from build123d import *

# Parameters (mm, degrees)
SKETCH2_R           = 57.15
SKETCH2_R_2         = 50.8
BOSS_EXTRUDE1_DEPTH = 101.6
SKETCH4_R           = 57.15
SKETCH4_R_2         = 50.8
BOSS_EXTRUDE2_DEPTH = 1.016
SKETCH5_R           = 1.27
CUT_EXTRUDE2_DEPTH  = 14.732


with BuildPart() as part:
    # Sketch2 → Boss-Extrude1 (new body)
    with BuildSketch(Plane(origin=(0, 0, 0), x_dir=(1, 0, 0), z_dir=(0, 1, 0))):
        with Locations(Location((0, 0, 0), (0, 0, 270))):
            Circle(SKETCH2_R)
        with Locations(Location((0, 0, 0), (0, 0, 270))):
            Circle(SKETCH2_R_2, mode=Mode.SUBTRACT)
    extrude(amount=BOSS_EXTRUDE1_DEPTH)

    # Sketch4 → Boss-Extrude2 (add)
    # profile 1 of 2: a face of its own
    with BuildSketch(Plane(origin=(0, 101.6, 0), x_dir=(1, 0, 0), z_dir=(0, 1, 0))):
        with Locations(Location((0, 0, 0), (0, 0, 270))):
            Circle(SKETCH4_R)
        with Locations(Location((0, 0, 0), (0, 0, 172.649423361))):
            Circle(SKETCH4_R_2, mode=Mode.SUBTRACT)
    # profile 2 of 2: a face of its own
    with BuildSketch(Plane(origin=(0, 101.6, 0), x_dir=(1, 0, 0), z_dir=(0, 1, 0))):
        with BuildLine():
            Line((-50.382520142, -6.499358748), (0, -6.499358748))
            Line((0, -6.499358748), (50.382520142, -6.499358748))
            ThreePointArc((50.382520142, -6.499358748), (50.695522599, -3.256376574), (50.8, 0))
            ThreePointArc((50.8, 0), (50.695522599, 3.256376574), (50.382520142, 6.499358748))
            Line((50.382520142, 6.499358748), (-50.382520142, 6.499358748))
            ThreePointArc((-50.382520142, 6.499358748), (-50.8, 0), (-50.382520142, -6.499358748))
        make_face()
    extrude(amount=BOSS_EXTRUDE2_DEPTH)

    # Sketch5 → Cut-Extrude2 (cut)
    with BuildSketch(Plane(origin=(0, 102.616, 0), x_dir=(1, 0, 0), z_dir=(0, 1, 0))):
        with Locations(Location((7.62, 0, 0), (0, 0, 270))):
            Circle(SKETCH5_R)
        with Locations(Location((-7.62, 0, 0), (0, 0, 270))):
            Circle(SKETCH5_R)
    extrude(amount=-CUT_EXTRUDE2_DEPTH, mode=Mode.SUBTRACT)


solid = part.part
Work out the finished part from the listing and answer in its coordinate system (mm). Coordinates: 2 decimals unless noted, no trailing zeros. Loops run counter-clockwise (first coordinate to the right, second up) from the corner with the lowest first, then second, coordinate; pieces in that order, holes last. Notation, with made-up numbers: M 79,41 L 100,41 A27 ccw 100,60 Z; hole C 79,81.25 d10. An arc over 180 degrees is marked long. Answer in a Markdown table with one row per item. Add a question column.
1. Flat-ended cylindrical pins translate along their axes: P1, Ø0.5, axis at x = 8, y = 102, coming from the +Z side; P2, Ø1.5, axis at x = -25, y = 76, coming from the -Z side; P3, Ø4, axis at x = -8.5, y = 14, coming from the -Z side. Find the tip coordinate at first contact, or state that the pin passes through.
2. Find section B-B, the plane z = 20.5. Write down the section's boundary in (x, y), then the cut area to 3 significant figures.
3. Find section A-A, the plane x = 0. Write down the section's boundary in (y, z).
4. The mould has two halves that part along Z. Classify faces 1 (the flat face through (-1, 101.6, 0)), 2 (the cylindrical face through (2.513, 50.59, -57.095)), 3 (the flat face through (-4, 102.616, 0)): pulls with the +Z half, pulls with the -Z half, needs draft (parallel to the pull), parting line crosses it, or undercut.
5. Consider L1, parallel to X at y = 102, z = 0; L2, parallel to X at y = 56, z = 0; L3, parallel to Z at x = 1, y = 60.5. Determine where each line is inside the solid, lowest interval first.
6. Find section C-C, the plane y = 30. Write down the section's boundary in (x, z).
7. Find section D-D, the plane x = 20.5. Write down the section's boundary in (y, z).
Reported:
| question | item | result |
|---|---|---|
| 1 | P1 | stops at z = 56.62 |
| 1 | P2 | stops at z = -51.75 |
| 1 | P3 | stops at z = -56.78 |
| 2 | outline | M -53.35,0 L -46.48,0 L -46.48,102.62 L -53.35,102.62 Z; M 46.48,0 L 53.35,0 L 53.35,102.62 L 46.48,102.62 Z |
| 2 | area | 1,410 mm^2 |
| 3 | outline | M 0,-57.15 L 102.62,-57.15 L 102.62,-50.8 L 0,-50.8 Z; M 0,50.8 L 102.62,50.8 L 102.62,57.15 L 0,57.15 Z; M 101.6,-6.5 L 102.62,-6.5 L 102.62,6.5 L 101.6,6.5 Z |
| 4 | face 1 | undercut |
| 4 | face 2 | parting line crosses it |
| 4 | face 3 | needs draft |
| 5 | L1 | x = -57.15 to -8.89, -6.35 to 6.35, 8.89 to 57.15 |
| 5 | L2 | x = -57.15 to -50.8, 50.8 to 57.15 |
| 5 | L3 | z = -57.14 to -50.79, 50.79 to 57.14 |
| 6 | outline | C 0,0 d114.3; hole C 0,0 d101.6 |
| 7 | outline | M 0,-53.35 L 102.62,-53.35 L 102.62,-46.48 L 0,-46.48 Z; M 0,46.48 L 102.62,46.48 L 102.62,53.35 L 0,53.35 Z; M 101.6,-6.5 L 102.62,-6.5 L 102.62,6.5 L 101.6,6.5 Z |
